Read the model definition and answer for the solid it produces. Units are mm, in the model's axes. A direction names the side the tool comes from. Give positions to 0.01 mm unless a question says otherwise; leave off trailing zeros. Loops run counter-clockwise (first coordinate to the right, second up) from the corner with the lowest first, then second, coordinate; pieces in that order, holes last. Notation, with made-up numbers: (-34, 0.25) - (-10, 0.25) arc R14 ccw to (-10, 12.25) - close; hole circle Ø8 at (-16.75, 3). An arc over 180 degrees is marked (long way). Put each result on its own line as item: value. Start each with the question number.
1. A cutting plane is placed at B-B, the plane y = -20. Determine the outline of the cut face in (x, z), plus the area to 3 significant figures.
2. For a pull along X with two mould halves and no side action, classify faces 4 (the flat face through (0, -5, -2)), 5 (the cylindrical face through (4.2, -0.6, 2.5)), 6 (the cylindrical face through (4.805, -18.513, -2.465)), 7 (the flat face through (10, -10, 0)) as released by +X, released by -X, zero draft, split by the parting line, or undercut.
3. Consider L1, parallel to Y at x = 5, z = -1.95; L2, parallel to Y at x = -5, z = 2.3; L3, parallel to Z at x = 9, y = 1. Determine where each line is inside the solid, lowest interval first. Write a range as from..to.
4. For faces 1 (the flat face through (0, 0, 0)), 2 (the flat face through (0, -20, 0)), 3 (the cylindrical face through (-5.8, -0.6, 2.5)), determine the directions among +Z, -Z, +X, -X, +Y, -Y from which every point of the face is accessible in a straight line to the end or side of a thin tool.
5. A cutting plane is placed at A-A, the plane x = 5. Determine the outline of the cut face in (y, z), plus the area to 3 significant figures.
6. A cutting plane is placed at D-D, the plane x = -7.75. Determine the outline of the cut face in (y, z), plus the area to 3 significant figures.
7. A cutting plane is placed at C-C, the plane z = -1. Determine the outline of the cut face in (x, y), plus the area to 3 significant figures.
8. Given pin 1 Ø3 at (x, y) = (1, -18) entering from +Z; pin 2 Ø5 at (x, y) = (-1, -1) entering from -Z; pin 3 Ø2.5 at (x, z) = (3, 3.5) entering from -Y; pin 4 Ø1.2 at (x, y) = (-5, 0) entering from +Z, each flat-ended and moving along its own axis, determine where each tip first touches the part or whether it passes through.
```python
from build123d import *

# Parameters (mm, degrees)
SKETCH1_W           = 20
SKETCH1_H           = 10
BOSS_EXTRUDE1_DEPTH = 5
SKETCH2_W           = 20
SKETCH2_H           = 5
BOSS_EXTRUDE2_DEPTH = 10
SKETCH3_W           = 20
SKETCH3_H           = 10
BOSS_EXTRUDE3_DEPTH = 5
SKETCH5_R           = 1
CUT_EXTRUDE1_DEPTH  = 10
SKETCH7_W           = 20
SKETCH7_H           = 5
BOSS_EXTRUDE5_DEPTH = 10
SKETCH8_R           = 1.5
CUT_EXTRUDE3_DEPTH  = 10


with BuildPart() as part:
    # Sketch1 → Boss-Extrude1 (new body)
    with BuildSketch(Plane.XY):
        Rectangle(SKETCH1_W, SKETCH1_H)
    extrude(amount=BOSS_EXTRUDE1_DEPTH)

    # Sketch2 → Boss-Extrude2 (add)
    with BuildSketch(Plane.XZ.offset(5)):
        with Locations((0, 2.5)):
            Rectangle(SKETCH2_W, SKETCH2_H)
    extrude(amount=BOSS_EXTRUDE2_DEPTH)

    # Sketch3 → Boss-Extrude3 (add)
    with BuildSketch(Plane(origin=(0, 0, 0), x_dir=(-1, 0, 0), z_dir=(0, 0, -1))):
        with Locations((0, -10)):
            Rectangle(SKETCH3_W, SKETCH3_H)
    extrude(amount=BOSS_EXTRUDE3_DEPTH)

    # Sketch5 → Cut-Extrude1 (cut)
    with BuildSketch(Plane.XY.offset(5)):
        with Locations((-5, 0)):
            Circle(SKETCH5_R)
        with Locations((5, 0)):
            Circle(SKETCH5_R)
    extrude(amount=-CUT_EXTRUDE1_DEPTH, mode=Mode.SUBTRACT)

    # Sketch7 → Boss-Extrude5 (add)
    with BuildSketch(Plane.XZ.offset(15)):
        with Locations((0, -2.5)):
            Rectangle(SKETCH7_W, SKETCH7_H)
    extrude(amount=BOSS_EXTRUDE5_DEPTH)

    # Sketch8 → Cut-Extrude3 (cut)
    with BuildSketch(Plane.XY):
        with Locations((-5, -20)):
            Circle(SKETCH8_R)
        with Locations((5, -20)):
            Circle(SKETCH8_R)
    extrude(amount=-CUT_EXTRUDE3_DEPTH, mode=Mode.SUBTRACT)


solid = part.part
```
Return value:
1. outline: (-10, -5) - (-6.5, -5) - (-6.5, 0) - (-10, 0) - close; (-3.5, -5) - (3.5, -5) - (3.5, 0) - (-3.5, 0) - close; (6.5, -5) - (10, -5) - (10, 0) - (6.5, 0) - close
1. area: 70.0 mm2
2. face 4: zero draft
2. face 5: undercut
2. face 6: undercut
2. face 7: released by +X
3. L1: y = -25..-21.5, -18.5..-5
3. L2: y = -15..-1, 1..5
3. L3: z = 0..5
4. face 1: -Z, +X, -X, +Y
4. face 2: +Z, +X, -X, -Y
4. face 3: +Z, -Z
5. outline: (-25, -5) - (-21.5, -5) - (-21.5, 0) - (-25, 0) - close; (-18.5, -5) - (-5, -5) - (-5, 0) - (-1, 0) - (-1, 5) - (-15, 5) - (-15, 0) - (-18.5, 0) - close; (1, 0) - (5, 0) - (5, 5) - (1, 5) - close
5. area: 175 mm2
6. outline: (-25, -5) - (-5, -5) - (-5, 0) - (5, 0) - (5, 5) - (-15, 5) - (-15, 0) - (-25, 0) - close
6. area: 200 mm2
7. outline: (-10, -25) - (10, -25) - (10, -5) - (-10, -5) - close; hole circle Ø3 at (-5, -20); hole circle Ø3 at (5, -20)
7. area: 386 mm2
8. pin 1: stops at z = 0
8. pin 2: stops at z = 0
8. pin 3: stops at y = -15
8. pin 4: passes through
